Autodesk Fusion 360 part; units mm, degrees
sketch "back" plane through (0, 0, 0) normal (0, 1, 0) x (1, 0, 0)
  arc A0 (-49, 26.4274) -> (-48.5607, 25.3667) centre (-47.5, 26.4274) ccw
  line L0 (-46, -19.363) -> (-54, -19.363)
  line L1 (-54.4393, -15.4237) -> (-73.3345, 3.4715)
  arc A1 (-48.5607, 29.2454) -> (-49, 28.1847) centre (-47.5, 28.1847) ccw
  line L2 (-48.5607, 25.3667) -> (-26.6655, 3.4715)
  arc A2 (-54, -16.4843) -> (-54.4393, -15.4237) centre (-55.5, -16.4843) ccw
  arc A3 (-51.4393, 25.3667) -> (-51, 26.4274) centre (-52.5, 26.4274) ccw
  arc A4 (-54.4393, 70.0358) -> (-54, 71.0964) centre (-55.5, 71.0964) ccw
  line L3 (-73.1931, 51.1406) -> (-54.3686, 69.965)
  arc A5 (-54.3686, 69.965) -> (-53.9, 71.0964) centre (-55.5, 71.0964) ccw
  line L4 (-53.9, -19.263) -> (-53.9, -16.4843)
  line L5 (-45.5607, 70.0358) -> (-26.6655, 51.1406)
  line L6 (-51, 26.4274) -> (-51, 28.1847)
  line L7 (-46.1, 73.8751) -> (-46.1, 71.0964)
  line L8 (-46.1, -16.4843) -> (-46.1, -19.263)
  arc A6 (-46, 71.0964) -> (-45.5607, 70.0358) centre (-44.5, 71.0964) ccw
  arc A7 (-45.5607, -15.4237) -> (-46, -16.4843) centre (-44.5, -16.4843) ccw
  line L9 (-54, 71.0964) -> (-54, 73.9751)
  arc A8 (-51, 28.1847) -> (-51.4393, 29.2454) centre (-52.5, 28.1847) ccw
  line L10 (-46, 73.9751) -> (-46, 71.0964)
  line L11 (-26.6655, 3.4715) -> (-45.5607, -15.4237)
  line L12 (-45.6314, 69.965) -> (-26.8069, 51.1406)
  arc A9 (-50.9, 28.1847) -> (-51.3686, 29.3161) centre (-52.5, 28.1847) ccw
  line L13 (-46, -16.4843) -> (-46, -19.363)
  line L14 (-54, -19.363) -> (-54, -16.4843)
  line L15 (-54, 73.9751) -> (-46, 73.9751)
  line L16 (-26.6655, 51.1406) -> (-48.5607, 29.2454)
  line L17 (-51.4393, 29.2454) -> (-73.3345, 51.1406)
  line L18 (-54.3686, -15.353) -> (-73.1931, 3.4715)
  arc A10 (-48.6314, 29.3161) -> (-49.1, 28.1847) centre (-47.5, 28.1847) ccw
  line L19 (-73.3345, 3.4715) -> (-51.4393, 25.3667)
  arc A11 (-51.3686, 25.296) -> (-50.9, 26.4274) centre (-52.5, 26.4274) ccw
  arc A12 (-49.1, 26.4274) -> (-48.6314, 25.296) centre (-47.5, 26.4274) ccw
  line L20 (-50.9, 26.4274) -> (-50.9, 28.1847)
  line L21 (-73.3345, 51.1406) -> (-54.4393, 70.0358)
  line L22 (-53.9, 71.0964) -> (-53.9, 73.8751)
  line L23 (-49, 28.1847) -> (-49, 26.4274)
  arc A13 (-46.1, 71.0964) -> (-45.6314, 69.965) centre (-44.5, 71.0964) ccw
  line L24 (-49.1, 28.1847) -> (-49.1, 26.4274)
  arc A14 (-45.6314, -15.353) -> (-46.1, -16.4843) centre (-44.5, -16.4843) ccw
  line L25 (-26.8069, 3.4715) -> (-45.6314, -15.353)
  arc A15 (-53.9, -16.4843) -> (-54.3686, -15.353) centre (-55.5, -16.4843) ccw
  line L26 (-26.8069, 51.1406) -> (-48.6314, 29.3161)
  line L27 (-73.1931, 3.4715) -> (-51.3686, 25.296)
  line L28 (-51.3686, 29.3161) -> (-73.1931, 51.1406)
  line L29 (-48.6314, 25.296) -> (-26.8069, 3.4715)
  line L30 (-46.1, -19.263) -> (-53.9, -19.263)
  line L31 (-53.9, 73.8751) -> (-46.1, 73.8751)
extrude "Extrude1" add sketch "back" along normal blind 2 contours L3 A5 L4 L7 L8 L12 A9 L18 A10 A11 A12 L20 L22 A13 L24 A14 L25 A15 L26 L27 L28 L29 L30 L31
Could you check a few things on this model? Use its own coordinates, in mm. A direction names the side the tool comes from. Give positions to 0.01 mm unless a question says otherwise; leave off trailing zeros. Loops run counter-clockwise (first coordinate to the right, second up) from the corner with the lowest first, then second, coordinate; pieces in that order, holes last. Notation, with made-up numbers: (27.5, 25.25) - (86.5, 25.25) arc R12 cw to (86.5, 43.25) - close; hole circle Ø10 at (-18.5, -25). An arc over 180 degrees is marked (long way). Answer in a Markdown table with one row per item. Add a question column.
Q1. If we section it at D-D (z = -15): List the corners of the cut face in (x, y) for me.
Q2. We'd pull the mould along Z, two halves only. Please class faces 1 (the face through (-63.65, 0.99, 6.07)), 2 (the face through (-36.351, 0.986, -60.685)), 3 (the face through (-50.9, 1, -27)): +Z half, -Z half, draft (parallel to the pull), parting line (faces both ways), or undercut.
Q3. For pin 1 (1 mm diameter, centred on y = 1, z = -73, fed in from -X); pin 2 (2 mm diameter, centred on x = -65, z = -42, fed in from +Y); pin 3 (0.6 mm diameter, centred on y = 1.5, z = 18.5, fed in from +X); pin 4 (0.5 mm diameter, centred on y = 1, z = -27, fed in from -X), each with a flat end and sliding along its axis, tell me the tip position at first contact or that it passes through.
Q4. If we section it at A-A (x = -47): List the corners of the cut face in (y, z) for me.
Q5. Which directions (+Z, -Z, +X, -X, +Y, -Y) give clear straight access to the entire face, cutting with the end or side of a thin tool? Please do faces 4 (the face through (-37.57, 0.99, -40.38)), 5 (the face through (-46.1, 1, -73)), 6 (the face through (-53.9, 1, -72)).
Q6. If we section it at B-B (y = 0.9): List the corners of the cut face in (x, z) for me (1 decimal).
Q7. If we section it at C-C (x = -56.5): List the corners of the cut face in (y, z) for me.
Q8. Please list where these lines run through material, in increasing order: L1, parallel to Z at x = -38, y = 0.7; L2, parallel to Z at x = -68, y = 0.35; L3, parallel to X at y = 0.6, z = -27. Write a range as from..to.
The answers:
| question | item | result |
|---|---|---|
| 1 | outline | (-61.66, 0) - (-38.34, 0) - (-38.34, 2) - (-61.66, 2) - close |
| 2 | face 1 | +Z half |
| 2 | face 2 | -Z half |
| 2 | face 3 | undercut |
| 3 | pin 1 | stops at x = -53.9 |
| 3 | pin 2 | stops at y = 2 |
| 3 | pin 3 | stops at x = -46.1 |
| 3 | pin 4 | stops at x = -50.9 |
| 4 | outline | (0, -73.88) - (2, -73.88) - (2, -30.95) - (0, -30.95) - close; (0, -23.66) - (2, -23.66) - (2, 19.26) - (0, 19.26) - close |
| 5 | face 4 | +X, +Y, -Y |
| 5 | face 5 | -Z, +X, +Y, -Y |
| 5 | face 6 | -Z, -X, +Y, -Y |
| 6 | outline | (-73.2, -51.1) - (-54.4, -70) arc R1.6 cw to (-53.9, -71.1) - (-53.9, -73.9) - (-46.1, -73.9) - (-46.1, -71.1) arc R1.6 cw to (-45.6, -70) - (-26.8, -51.1) - (-48.6, -29.3) arc R1.6 cw to (-49.1, -28.2) - (-49.1, -26.4) arc R1.6 cw to (-48.6, -25.3) - (-26.8, -3.5) - (-45.6, 15.4) arc R1.6 cw to (-46.1, 16.5) - (-46.1, 19.3) - (-53.9, 19.3) - (-53.9, 16.5) arc R1.6 cw to (-54.4, 15.4) - (-73.2, -3.5) - (-51.4, -25.3) arc R1.6 cw to (-50.9, -26.4) - (-50.9, -28.2) arc R1.6 cw to (-51.4, -29.3) - close |
| 7 | outline | (0, -67.83) - (2, -67.83) - (2, -34.45) - (0, -34.45) - close; (0, -20.16) - (2, -20.16) - (2, 13.22) - (0, 13.22) - close |
| 8 | L1 | z = -62.33..-39.95, -14.66..7.72 |
| 8 | L2 | z = -56.33..-45.95, -8.66..1.72 |
| 8 | L3 | x = -50.9..-49.1 |
